CAD build for the part. Positions are in the model's coordinates, mm. A direction names the side the tool comes from. Give positions to 0.01 mm unless a question says otherwise; leave off trailing zeros. Order: outer loops, then holes, each group sorted by start corner. A loop starts at its lowest first (then second) coordinate and runs counter-clockwise, first axis right, second up.
```python
from build123d import *

# Parameters (mm, degrees)
EXTRUDE_1_DEPTH          = 170
SKETCH_2_R               = 60
CUT_EXTRUDE_1_DEPTH      = 180
CUT_EXTRUDE_2_DEPTH      = 313.955268369
CUT_EXTRUDE_2_DEPTH_BACK = 313.955268369
SKETCH_3_R               = 17.5
FILLET_1_R               = 70
FILLET_2_R               = 5
FILLET_3_R               = 10
SKETCH_6_R               = 30
CUT_EXTRUDE_6_DEPTH      = 39
SKETCH_10_R              = 2.5
CUT_EXTRUDE_10_DEPTH     = 10
CUT_EXTRUDE_START        = -4
SKETCH_11_R              = 6
SKETCH_11_R_2            = 2.5
CUT_EXTRUDE_11_DEPTH     = 4
SKETCH_12_R              = 2.75
CUT_EXTRUDE_12_DEPTH     = 10
EXTRUDE_START            = 10.5
SKETCH_14_R              = 27.5
SKETCH_14_R_2            = 17.5
EXTRUDE_2_DEPTH          = 10.5
SKETCH_13_R              = 2.25
CUT_EXTRUDE_13_DEPTH     = 15


with BuildPart() as part:
    # 草图1 → 凸台-拉伸1 (new body)
    with BuildSketch(Plane.XY):
        Polygon((-180, 0), (0, 0), (0, -175), (8, -175), (8, 8), (-180, 8), (-188, 8), (-188, -175), (-180, -175), align=None)
    extrude(amount=EXTRUDE_1_DEPTH)

    # 草图2 → 切除-拉伸1 (cut)
    with BuildSketch(Plane(origin=(0, 8, 0), x_dir=(1, 0, 0), z_dir=(0, 1, 0))):
        with Locations(Location((-90, -85, 0), (0, 0, 180))):
            Circle(SKETCH_2_R)
    extrude(amount=-CUT_EXTRUDE_1_DEPTH, mode=Mode.SUBTRACT)

    # 草图3 → 切除-拉伸2 (cut, two sides: drawn at the far end of the back side and taken through both)
    with BuildSketch(Plane(origin=(8, 0, 0), x_dir=(0, 0, -1), z_dir=(1, 0, 0)).offset(-CUT_EXTRUDE_2_DEPTH_BACK)):
        with Locations(Location((-85, -95, 0), (0, 0, 90))):
            Circle(SKETCH_3_R)
    extrude(amount=CUT_EXTRUDE_2_DEPTH + CUT_EXTRUDE_2_DEPTH_BACK, mode=Mode.SUBTRACT)

    # 圆角1
    fillet_1_edges = [part.edges().sort_by_distance(p)[0] for p in [
        (4, -175, 0),
        (4, -175, 170),
        (-184, -175, 170),
        (-184, -175, 0),
    ]]
    fillet(fillet_1_edges, radius=FILLET_1_R)

    # 圆角2
    fillet_2_edges = [part.edges().sort_by_distance(p)[0] for p in [
        (0, 0, 85),
        (-180, 0, 85),
    ]]
    fillet(fillet_2_edges, radius=FILLET_2_R)

    # 圆角3
    fillet_3_edges = [part.edges().sort_by_distance(p)[0] for p in [
        (-188, 8, 85),
        (8, 8, 85),
    ]]
    fillet(fillet_3_edges, radius=FILLET_3_R)

    # 草图6 → 切除-拉伸6 (cut)
    with BuildSketch(Plane.ZY.offset(188)):
        with Locations(Location((85, -95, 0), (0, 0, 270))):
            Circle(SKETCH_6_R)
    extrude(amount=-CUT_EXTRUDE_6_DEPTH, mode=Mode.SUBTRACT)

    # 草图10 → 切除-拉伸10 (cut)
    with BuildSketch(Plane.XZ):
        with Locations(Location((-55.742253069, 158.674753309, 0), (0, 0, 270))):
            Circle(SKETCH_10_R)
        with Locations(Location((-32.485217492, 142.390001682, 0), (0, 0, 270))):
            Circle(SKETCH_10_R)
        with Locations(Location((-9.066918551, 92.169297536, 0), (0, 0, 270))):
            Circle(SKETCH_10_R)
        with Locations(Location((-11.541409366, 63.885738097, 0), (0, 0, 270))):
            Circle(SKETCH_10_R)
        with Locations(Location((-16.325246691, 50.742253069, 0), (0, 0, 270))):
            Circle(SKETCH_10_R)
        with Locations(Location((-32.609998318, 27.485217492, 0), (0, 0, 270))):
            Circle(SKETCH_10_R)
        with Locations(Location((-124.257746931, 11.325246691, 0), (0, 0, 270))):
            Circle(SKETCH_10_R)
        with Locations(Location((-147.514782508, 27.609998318, 0), (0, 0, 270))):
            Circle(SKETCH_10_R)
        with Locations(Location((-170.933081449, 77.830702464, 0), (0, 0, 270))):
            Circle(SKETCH_10_R)
        with Locations(Location((-168.458590634, 106.114261903, 0), (0, 0, 270))):
            Circle(SKETCH_10_R)
        with Locations(Location((-163.674753309, 119.257746931, 0), (0, 0, 270))):
            Circle(SKETCH_10_R)
        with Locations(Location((-147.390001682, 142.514782508, 0), (0, 0, 270))):
            Circle(SKETCH_10_R)
    extrude(amount=-CUT_EXTRUDE_10_DEPTH, mode=Mode.SUBTRACT)

    # 草图11 → 切除-拉伸11 (cut)
    # profile 1 of 12: a face of its own
    with BuildSketch(Plane(origin=(0, 8, 0), x_dir=(1, 0, 0), z_dir=(0, 1, 0)).offset(CUT_EXTRUDE_START)):
        with Locations(Location((-32.485217492, -142.390001682, 0), (0, 0, 180))):
            Circle(SKETCH_11_R)
        with Locations(Location((-32.485217492, -142.390001682, 0), (0, 0, 90))):
            Circle(SKETCH_11_R_2, mode=Mode.SUBTRACT)
    # profile 2 of 12: a face of its own
    with BuildSketch(Plane(origin=(0, 8, 0), x_dir=(1, 0, 0), z_dir=(0, 1, 0)).offset(CUT_EXTRUDE_START)):
        with Locations(Location((-55.742253069, -158.674753309, 0), (0, 0, 180))):
            Circle(SKETCH_11_R)
        with Locations(Location((-55.742253069, -158.674753309, 0), (0, 0, 90))):
            Circle(SKETCH_11_R_2, mode=Mode.SUBTRACT)
    # profile 3 of 12: a face of its own
    with BuildSketch(Plane(origin=(0, 8, 0), x_dir=(1, 0, 0), z_dir=(0, 1, 0)).offset(CUT_EXTRUDE_START)):
        with Locations(Location((-147.390001682, -142.514782508, 0), (0, 0, 180))):
            Circle(SKETCH_11_R)
        with Locations(Location((-147.390001682, -142.514782508, 0), (0, 0, 90))):
            Circle(SKETCH_11_R_2, mode=Mode.SUBTRACT)
    # profile 4 of 12: a face of its own
    with BuildSketch(Plane(origin=(0, 8, 0), x_dir=(1, 0, 0), z_dir=(0, 1, 0)).offset(CUT_EXTRUDE_START)):
        with Locations(Location((-163.674753309, -119.257746931, 0), (0, 0, 180))):
            Circle(SKETCH_11_R)
        with Locations(Location((-163.674753309, -119.257746931, 0), (0, 0, 90))):
            Circle(SKETCH_11_R_2, mode=Mode.SUBTRACT)
    # profile 5 of 12: a face of its own
    with BuildSketch(Plane(origin=(0, 8, 0), x_dir=(1, 0, 0), z_dir=(0, 1, 0)).offset(CUT_EXTRUDE_START)):
        with Locations(Location((-168.458590634, -106.114261903, 0), (0, 0, 180))):
            Circle(SKETCH_11_R)
        with Locations(Location((-168.458590634, -106.114261903, 0), (0, 0, 90))):
            Circle(SKETCH_11_R_2, mode=Mode.SUBTRACT)
    # profile 6 of 12: a face of its own
    with BuildSketch(Plane(origin=(0, 8, 0), x_dir=(1, 0, 0), z_dir=(0, 1, 0)).offset(CUT_EXTRUDE_START)):
        with Locations(Location((-170.933081449, -77.830702464, 0), (0, 0, 180))):
            Circle(SKETCH_11_R)
        with Locations(Location((-170.933081449, -77.830702464, 0), (0, 0, 90))):
            Circle(SKETCH_11_R_2, mode=Mode.SUBTRACT)
    # profile 7 of 12: a face of its own
    with BuildSketch(Plane(origin=(0, 8, 0), x_dir=(1, 0, 0), z_dir=(0, 1, 0)).offset(CUT_EXTRUDE_START)):
        with Locations(Location((-147.514782508, -27.609998318, 0), (0, 0, 180))):
            Circle(SKETCH_11_R)
        with Locations(Location((-147.514782508, -27.609998318, 0), (0, 0, 90))):
            Circle(SKETCH_11_R_2, mode=Mode.SUBTRACT)
    # profile 8 of 12: a face of its own
    with BuildSketch(Plane(origin=(0, 8, 0), x_dir=(1, 0, 0), z_dir=(0, 1, 0)).offset(CUT_EXTRUDE_START)):
        with Locations(Location((-124.257746931, -11.325246691, 0), (0, 0, 180))):
            Circle(SKETCH_11_R)
        with Locations(Location((-124.257746931, -11.325246691, 0), (0, 0, 90))):
            Circle(SKETCH_11_R_2, mode=Mode.SUBTRACT)
    # profile 9 of 12: a face of its own
    with BuildSketch(Plane(origin=(0, 8, 0), x_dir=(1, 0, 0), z_dir=(0, 1, 0)).offset(CUT_EXTRUDE_START)):
        with Locations(Location((-32.609998318, -27.485217492, 0), (0, 0, 180))):
            Circle(SKETCH_11_R)
        with Locations(Location((-32.609998318, -27.485217492, 0), (0, 0, 90))):
            Circle(SKETCH_11_R_2, mode=Mode.SUBTRACT)
    # profile 10 of 12: a face of its own
    with BuildSketch(Plane(origin=(0, 8, 0), x_dir=(1, 0, 0), z_dir=(0, 1, 0)).offset(CUT_EXTRUDE_START)):
        with Locations(Location((-16.325246691, -50.742253069, 0), (0, 0, 180))):
            Circle(SKETCH_11_R)
        with Locations(Location((-16.325246691, -50.742253069, 0), (0, 0, 90))):
            Circle(SKETCH_11_R_2, mode=Mode.SUBTRACT)
    # profile 11 of 12: a face of its own
    with BuildSketch(Plane(origin=(0, 8, 0), x_dir=(1, 0, 0), z_dir=(0, 1, 0)).offset(CUT_EXTRUDE_START)):
        with Locations(Location((-11.541409366, -63.885738097, 0), (0, 0, 180))):
            Circle(SKETCH_11_R)
        with Locations(Location((-11.541409366, -63.885738097, 0), (0, 0, 90))):
            Circle(SKETCH_11_R_2, mode=Mode.SUBTRACT)
    # profile 12 of 12: a face of its own
    with BuildSketch(Plane(origin=(0, 8, 0), x_dir=(1, 0, 0), z_dir=(0, 1, 0)).offset(CUT_EXTRUDE_START)):
        with Locations(Location((-9.066918551, -92.169297536, 0), (0, 0, 180))):
            Circle(SKETCH_11_R)
        with Locations(Location((-9.066918551, -92.169297536, 0), (0, 0, 90))):
            Circle(SKETCH_11_R_2, mode=Mode.SUBTRACT)
    extrude(amount=CUT_EXTRUDE_11_DEPTH, mode=Mode.SUBTRACT)

    # 草图12 → 切除-拉伸12 (cut)
    with BuildSketch(Plane.ZY.offset(188)):
        with Locations(Location((94.058666579, -128.80740392, 0), (0, 0, 270))):
            Circle(SKETCH_12_R)
        with Locations(Location((75.941333421, -128.80740392, 0), (0, 0, 270))):
            Circle(SKETCH_12_R)
        with Locations(Location((60.251262658, -119.748737342, 0), (0, 0, 270))):
            Circle(SKETCH_12_R)
        with Locations(Location((51.19259608, -104.058666579, 0), (0, 0, 270))):
            Circle(SKETCH_12_R)
        with Locations(Location((51.19259608, -85.941333421, 0), (0, 0, 270))):
            Circle(SKETCH_12_R)
        with Locations(Location((60.251262658, -70.251262658, 0), (0, 0, 270))):
            Circle(SKETCH_12_R)
        with Locations(Location((75.941333421, -61.19259608, 0), (0, 0, 270))):
            Circle(SKETCH_12_R)
        with Locations(Location((94.058666579, -61.19259608, 0), (0, 0, 270))):
            Circle(SKETCH_12_R)
        with Locations(Location((109.748737342, -70.251262658, 0), (0, 0, 270))):
            Circle(SKETCH_12_R)
        with Locations(Location((118.80740392, -85.941333421, 0), (0, 0, 270))):
            Circle(SKETCH_12_R)
        with Locations(Location((118.80740392, -104.058666579, 0), (0, 0, 270))):
            Circle(SKETCH_12_R)
        with Locations(Location((109.748737342, -119.748737342, 0), (0, 0, 270))):
            Circle(SKETCH_12_R)
    extrude(amount=-CUT_EXTRUDE_12_DEPTH, mode=Mode.SUBTRACT)

    # 草图14 → 凸台-拉伸2 (add)
    with BuildSketch(Plane(origin=(8, 0, 0), x_dir=(0, 0, -1), z_dir=(1, 0, 0)).offset(EXTRUDE_START)):
        with Locations(Location((-85, -95, 0), (0, 0, 270))):
            Circle(SKETCH_14_R)
        with Locations(Location((-85, -95, 0), (0, 0, 90))):
            Circle(SKETCH_14_R_2, mode=Mode.SUBTRACT)
    extrude(amount=-EXTRUDE_2_DEPTH)

    # 草图13 → 切除-拉伸13 (cut, symmetric)
    with BuildSketch(Plane(origin=(8, 0, 0), x_dir=(0, 0, -1), z_dir=(1, 0, 0))):
        with Locations(Location((-85, -72.5, 0), (0, 0, 90))):
            Circle(SKETCH_13_R)
        with Locations(Location((-69.090097423, -79.090097423, 0), (0, 0, 90))):
            Circle(SKETCH_13_R)
        with Locations(Location((-62.5, -95, 0), (0, 0, 90))):
            Circle(SKETCH_13_R)
        with Locations(Location((-69.090097423, -110.909902577, 0), (0, 0, 90))):
            Circle(SKETCH_13_R)
        with Locations(Location((-85, -117.5, 0), (0, 0, 90))):
            Circle(SKETCH_13_R)
        with Locations(Location((-100.909902577, -110.909902577, 0), (0, 0, 90))):
            Circle(SKETCH_13_R)
        with Locations(Location((-107.5, -95, 0), (0, 0, 90))):
            Circle(SKETCH_13_R)
        with Locations(Location((-100.909902577, -79.090097423, 0), (0, 0, 90))):
            Circle(SKETCH_13_R)
    extrude(amount=CUT_EXTRUDE_13_DEPTH, both=True, mode=Mode.SUBTRACT)


solid = part.part
```
Item 1: Two-plate mould, pull along X, no slides. Class faces 1 (the face through (18.5, -82, 72)), 2 (the face through (-188, -68, 65)), 3 (the face through (-184.06, -101.31, 51.31)), 4 (the face through (-32.375, 1.972, 144.888)): released by +X, released by -X, zero draft, split by the parting line, or undercut.
Item 2: Slice it at A-A (x = -90). Give the cut face in (y, z), and give its area (3 significant figures).
Item 3: Slice it at B-B (y = -42). Give the cut face in (x, z), and give its area (3 significant figures).
Item 4: Wall check: L1, parallel to X at y = -20, z = 59; L2, parallel to Z at x = 14.75, y = -95; L3, parallel to Y at x = -47.5, z = 26. Give the ranges that are in metal, low to high.
Item 5: Drop flat-ended pins along their axis: pin 1 Ø4.5 at (y, z) = (-70.25, 60.25) entering from +X; pin 2 Ø6 at (y, z) = (-95, 62.5) entering from -X; pin 3 Ø6.5 at (x, z) = (-168.46, 106.11) entering from -Y. Give the stop position or say it passes through.
Item 6: Tool access for faces 5 (the face through (-2, -1, 86)), 6 (the face through (-148.91, 1.97, 144.5)), 7 (the face through (-118.264, 5.972, 11.589)): list every direction of +Z, -Z, +X, -X, +Y, -Y with a clear straight run to the whole face (end or side of a thin tool).
A:
1. face 1: released by +X
1. face 2: released by -X
1. face 3: zero draft
1. face 4: undercut
2. outline: (0, 0) - (8, 0) - (8, 25) - (0, 25) - close; (0, 145) - (8, 145) - (8, 170) - (0, 170) - close
2. area: 400 mm2
3. outline: (-188, 0) - (-180, 0) - (-180, 170) - (-188, 170) - close; (0, 0) - (8, 0) - (8, 170) - (0, 170) - close
3. area: 2,720 mm2
4. L1: x = -188 to -180, 0 to 8
4. L2: z = 57.5 to 60.25, 64.75 to 67.5, 102.5 to 105.25, 109.75 to 112.5
4. L3: y = 0 to 8
5. pin 1: stops at x = 8
5. pin 2: stops at x = 0
5. pin 3: stops at y = 0
6. face 5: +Z, -Z, -Y
6. face 6: +Y, -Y
6. face 7: +Y
